Check sheet for the modelled part. Datum: model origin and axes. Units: mm. A direction names the side the tool comes from. Give positions to 0.01 mm unless a question says otherwise; leave off trailing zeros. Write each loop counter-clockwise with the first axis right and the second up, starting at its lowest first coordinate (ties: lowest second). Pieces come first, ordered by that corner, then holes.
Autodesk Inventor part; units mm, degrees
ref_plane "YZ Plane" through (0, 0, 0) normal (1, 0, 0) x (0, 1, 0)
ref_plane "XZ Plane" through (0, 0, 0) normal (0, 1, 0) x (-1, 0, 0)
ref_plane "XY Plane" through (0, 0, 0) normal (0, 0, 1) x (1, 0, 0)
sketch "Szkic8" plane through (0, 0, 0) normal (0, 1, 0) x (-1, 0, 0)
  circle A0 centre (0, 0) radius 64.5
  circle A1 centre (0, 0) radius 62.5
  dimension "d53" = 129
  dimension "d54" = 2
extrude "Wyciągnięcie proste2" add sketch "Szkic8" along normal mid plane 375
sketch "Szkic13" plane through (0, 0, 0) normal (0, 0, 1) x (1, 0, 0)
  circle A0 centre (0, 0) radius 25.5
  circle A1 centre (0, 0) radius 23.5
  dimension "d67" = 51
  dimension "d68" = 2
extrude "Wyciągnięcie proste6" add sketch "Szkic13" along normal blind 68.5
sketch "Szkic14" plane through (0, 0, 68.5) normal (0, 0, 1) x (1, 0, 0)
  circle A0 centre (0, 0) radius 23.5
extrude "Wyciągnięcie proste7" cut sketch "Szkic14" against normal blind 68.5
sketch "Szkic15" plane through (0, -187.5, 0) normal (0, -1, 0) x (1, 0, 0)
  circle A0 centre (0, 0) radius 62.5
extrude "Wyciągnięcie proste8" cut sketch "Szkic15" against normal blind 375
fillet "Zaokrąglenie3" radius 2 2 edges at (-0.0041, 25.5, 64.5) (0.0041, -25.5, 64.5)
fillet "Zaokrąglenie4" radius 4 2 edges at (-0.0002, -23.5, 62.5) (-0.0017, 23.5, 62.5)
equation "\"d53\" = OD"
equation "\"d54\" = THK"
equation "\"d55\" = L1"
equation "\"d67\" = OD2"
equation "\"d68\" = THK"
equation "\"d69\" = L2"
equation "\"d71\" = L2"
equation "\"d73\" = L1"
equation "\"d75\" = THK"
equation "\"d76\" = 2 * THK"
equation "\"SzerokośćGięciaPodcięcia\" = Grubość"
equation "\"RozmiarPodcięciaNarożnika\" = 4 * Grubość"
equation "\"PromieńPrzejścia\" = PromieńGięcia"
equation "\"Rozmiar_promienia_Jacobiego\" = PromieńGięcia"
equation "\"Wielk_odstępu\" = Grubość"
equation "\"d2\" = PromieńGięcia"
equation "\"d23\" = PromieńGięcia"
equation "\"OD\" = 129"
equation "\"THK\" = 2"
equation "\"L1\" = 375"
equation "\"L2\" = 68.5"
equation "\"OD2\" = 51"
properties part number "Trójnik red. krótki  Ø129 51 129 s=2 L=375" material "304"
1) Sectioned sample at C-C on y = -146. Record the boundary of the cut face in (x, z), then the cut area to 3 significant figures.
2) Scan lines: L1, parallel to Z at x = 0, y = -39.5; L2, parallel to X at y = 0, z = 62.5; L3, parallel to Y at x = 0, z = 64. Record each from-to range of solid material in increasing order.
3) Draft check along Z on faces 3 (the cylindrical face through (13.549, 2.625, -61.014)), 4 (the flat face through (34, 187.5, 53)), 5 (the flat face through (11, -21, 68.5)). Enter one of: +Z half, -Z half, draft (parallel to the pull), parting line (faces both ways), or undercut.
4) Gauge pin test, flat ends, axial feed: pin 1 (6 mm diameter, centred on x = 3.5, y = -55.5, fed in from -Z); pin 2 (12 mm diameter, centred on y = -33, z = -18, fed in from +X); pin 3 (1 mm diameter, centred on y = -13, z = 47.5, fed in from -X). Record the tip position at first contact, or that the pin passes through.
5) Sectioned sample at A-A on z = 0. Record the boundary of the cut face in (x, y), then the cut area to 3 significant figures.
6) Access from +Z, -Z, +X, -X, +Y, -Y to the whole of each face (thin tool, end or side, straight path). Record for faces 1 (the cylindrical face through (-5.094, 22.941, 67.118)), 2 (the flat face through (34, -187.5, 53)).
7) Sectioned sample at D-D on x = 0. Give the number of separate pieces and of enclosed holes in the cut face, then the cut area to 3 significant figures.
8) Sectioned sample at B-B on x = -35. Record the boundary of the cut face in (y, z).
Answers below:
1. outline: circle Ø129 at (0, 0); hole circle Ø125 at (0, 0)
1. area: 798 mm2
2. L1: z = -64.5 to -62.5, 62.5 to 64.5
2. L2: x = -25.5 to -23.5, 23.5 to 25.5
2. L3: y = -187.5 to -24.38, 24.38 to 187.5
3. face 3: undercut
3. face 4: draft
3. face 5: +Z half
4. pin 1: stops at z = -64.5
4. pin 2: stops at x = 63.37
4. pin 3: stops at x = -44.17
5. outline: (-64.5, -187.5) - (-62.5, -187.5) - (-62.5, 187.5) - (-64.5, 187.5) - close; (62.5, -187.5) - (64.5, -187.5) - (64.5, 187.5) - (62.5, 187.5) - close
5. area: 1,500 mm2
6. face 1: +Z
6. face 2: +Z, -Z, +X, -X, -Y
7. separate pieces: 3
7. enclosed holes: 0
7. area: 1,420 mm2
8. outline: (-187.5, -54.18) - (187.5, -54.18) - (187.5, -51.78) - (-187.5, -51.78) - close; (-187.5, 51.78) - (187.5, 51.78) - (187.5, 54.18) - (-187.5, 54.18) - close
